from build123d import *

# Parameters (mm, degrees)
F1_DEPTH = 304.8
F2_R     = 6.35
F3_DEPTH = 6.35
F4_R     = 6.35
F5_DEPTH = 6.35
F6_R     = 6.35
F7_DEPTH = 6.35


with BuildPart() as f1:
    # F0 (on Front) → F1 (new body)
    with BuildSketch(Plane.XZ):
        with BuildLine():
            Line((0, 50.8), (0, 0))
            Line((0, 0), (50.8, 0))
            ThreePointArc((50.8, 0), (48.940128, 4.490128), (44.45, 6.35))
            Line((44.45, 6.35), (12.7, 6.35))
            ThreePointArc((12.7, 6.35), (8.209872, 8.209872), (6.35, 12.7))
            Line((6.35, 12.7), (6.35, 44.45))
            ThreePointArc((6.35, 44.45), (4.490128, 48.940128), (0, 50.8))
        make_face()
    extrude(amount=-F1_DEPTH)

    # F2 (on face) → F3 (cut)
    with BuildSketch(Plane(origin=(0, 0, 0), x_dir=(0, -1, 0), z_dir=(-1, 0, 0))):
        with Locations((-38.1, 25.4)):
            Circle(F2_R)
    extrude(amount=-F3_DEPTH, mode=Mode.SUBTRACT)

    # F4 (on face) → F5 (cut)
    with BuildSketch(Plane(origin=(0, 0, 0), x_dir=(0, -1, 0), z_dir=(-1, 0, 0))):
        with Locations((-266.7, 25.4)):
            Circle(F4_R)
    extrude(amount=-F5_DEPTH, mode=Mode.SUBTRACT)

    # F6 (on face) → F7 (cut)
    with BuildSketch(Plane(origin=(0, 0, 0), x_dir=(0, -1, 0), z_dir=(-1, 0, 0))):
        with Locations((-152.4, 25.4)):
            Circle(F6_R)
    extrude(amount=-F7_DEPTH, mode=Mode.SUBTRACT)


solid = f1.part
Design review of the part built by this model. Coordinates are the model's own, in mm. A direction names the side the tool comes from. Round coordinates to 2 decimals unless told otherwise and drop trailing zeros. Write each loop counter-clockwise with the first axis right and the second up, starting at its lowest first coordinate (ties: lowest second). Pieces come first, ordered by that corner, then holes. Notation, with made-up numbers: (81, -28) - (90, -28) arc R12 cw to (90, -5) - close; hole circle Ø8 at (-12.75, 14.25). An arc over 180 degrees is marked (long way). Return JSON: item names as keys, results as strings. Group by question number.
Item 1: Insertion check: P1, Ø8, axis at x = 15.5, z = 13.5, coming from the -Y side; P2, Ø4, axis at x = 23, y = 72.5, coming from the +Z side; P3, Ø10, axis at y = 129.5, z = 10, coming from the +X side; P4, Ø3, axis at x = 15.5, y = 78, coming from the -Z side. Each pin has a flat end and moves straight along its axis. Give the tip position at first contact, or say it passes through.
Item 2: We need section C-C on y = 107.5. Write out the cut boundary in (x, z), and give its area (3 significant figures).
Item 3: The part is to be moulded in two halves that separate along Z. For faces 3 (the face through (3.131, 260.834, 22.968)), 4 (the face through (25, 150, 0)), 5 (the face through (3.131, 146.343, 27.307)), 6 (the face through (29, 150, 6.35)), say which applies: pulls with the +Z half, pulls with the -Z half, needs draft (parallel to the pull), parting line crosses it, or undercut.
Item 4: For probe 1 along Y at (x, z) = (3, 25); probe 2 along Y at (x, z) = (3.5, 23.5); probe 3 along X at (y, z) = (126.5, 35), list the stretches that pass through material, from the lowest coordinate up. Write a range as [from, to].
Item 5: We need section B-B on z = 25.4. Write out the cut boundary in (x, y).
Item 6: We need section D-D on x = 31. Write out the cut boundary in (y, z), and give its area (3 significant figures).
Item 7: We need section A-A on y = 152.4. Write out the cut boundary in (x, z).
Item 8: Machinability: for faces 1 (the face through (3.131, 32.234, 22.968)), 2 (the face through (6.35, 150, 32)), which of the approach directions +Z, -Z, +X, -X, +Y, -Y give a long, thin tool a straight path to every point of the face, cutting with its end or side? Answer none if there is none.
Model answer:
{
 "1": {"P1": "passes through", "P2": "stops at z = 6.35", "P3": "stops at x = 48.36", "P4": "stops at z = 0"},
 "2": {"outline": "(0, 0) - (50.8, 0) arc R6.35 ccw to (44.45, 6.35) - (12.7, 6.35) arc R6.35 cw to (6.35, 12.7) - (6.35, 44.45) arc R6.35 ccw to (0, 50.8) - close", "area": "596 mm²"},
 "3": {"face 3": "undercut", "face 4": "pulls with the -Z half", "face 5": "undercut", "face 6": "pulls with the +Z half"},
 "4": {"probe 1": "y = [0, 31.76], [44.44, 146.06], [158.74, 260.36], [273.04, 304.8]", "probe 2": "y = [0, 32.04], [44.16, 146.34], [158.46, 260.64], [272.76, 304.8]", "probe 3": "x = [0, 6.35]"},
 "5": {"outline": "(0, 0) - (6.35, 0) - (6.35, 31.75) - (0, 31.75) - close; (0, 44.45) - (6.35, 44.45) - (6.35, 146.05) - (0, 146.05) - close; (0, 158.75) - (6.35, 158.75) - (6.35, 260.35) - (0, 260.35) - close; (0, 273.05) - (6.35, 273.05) - (6.35, 304.8) - (0, 304.8) - close"},
 "6": {"outline": "(0, 0) - (304.8, 0) - (304.8, 6.35) - (0, 6.35) - close", "area": "1,940 mm²"},
 "7": {"outline": "(0, 0) - (50.8, 0) arc R6.35 ccw to (44.45, 6.35) - (12.7, 6.35) arc R6.35 cw to (6.35, 12.7) - (6.35, 19.05) - (0, 19.05) - close; (0, 31.75) - (6.35, 31.75) - (6.35, 44.45) arc R6.35 ccw to (0, 50.8) - close"},
 "8": {"face 1": "+X, -X", "face 2": "+Z, +X, +Y, -Y"}
}
